The model under review builds one solid part; all positions refer to its coordinate system, in mm. A direction names the side the tool comes from. Round coordinates to 2 decimals unless told otherwise and drop trailing zeros. Write each loop counter-clockwise with the first axis right and the second up, starting at its lowest first coordinate (ties: lowest second). Pieces come first, ordered by that corner, then holes. Notation, with made-up numbers: (-27.75, 73) -> (-21.75, 73) arc R19 ccw to (-21.75, 87) -> close; hole circle Ø6 at (81, 61). An arc over 180 degrees is marked (long way). Use CSV: the item, a comma, the result in double quotes. Start each with the question number.
1) For pin 1 Ø3 at (y, z) = (-23, 26.5) entering from -X; pin 2 Ø5 at (x, z) = (-10, -15) entering from +Y; pin 3 Ø6 at (x, y) = (11.5, 27.5) entering from -Z; pin 4 Ø6.5 at (x, y) = (6.4, -11.09) entering from -Z, all flat-tipped, find the tip position at first contact; note any pin that passes through.
2) Take a section at A-A, the plane y = -9.5. State how many separate pieces and enclosed holes the cut face has, then the cut area to 3 significant figures.
3) Wall thickness on probe 1 along Z at (x, y) = (6, -2.5); probe 2 along Z at (x, y) = (-1, -24.5); probe 3 along X at (y, z) = (-18, 4.5): over which ranges is each line inside the solid? List them lowest first. Write a range as [from, to].
4) Machinability: for faces 1 (the face through (-0.867, 3.905, -20.514)), 2 (the face through (-4.336, -19.524, -3.853)), 3 (the face through (-4.336, -19.524, 44.854)), which of the approach directions +Z, -Z, +X, -X, +Y, -Y give a long, thin tool a straight path to every point of the face, cutting with its end or side? Answer none if there is none.
5) Mouldability with a two-part tool opening along X and no side actions: class faces 4 (the face through (15.213, -4.791, -23.021)), 5 (the face through (-10, 0, -23)), 6 (the face through (3, 3, -19.5)), 7 (the face through (5.11, 8.6, -23.02)) as released by +X, released by -X, zero draft, split by the parting line, or undercut.
6) Take a section at B-B, the plane z = 17. Give the boundary of the cut face in (x, y).
from build123d import *

# Parameters (mm, degrees)
SKETCH_1_R          = 35.1
EXTRUDE_1_DEPTH     = 45.1
SKETCH_3_R          = 30
SKETCH_3_R_2        = 20
EXTRUDE_2_DEPTH     = 3.5
SKETCH_3_4_R        = 20
EXTRUDE_3_DEPTH     = 24.5
FILLET_1_R          = 5
FILLET_2_R          = 20
FILLET_3_R          = 1
SKETCH_6_R          = 2.8
CUT_EXTRUDE_1_DEPTH = 4
SKETCH_7_R          = 25
SKETCH_7_R_2        = 20
CUT_EXTRUDE_2_DEPTH = 0.5


with BuildPart() as part:
    # Sketch 1 → Extrude 1 (new body)
    with BuildSketch(Plane.XY):
        Circle(SKETCH_1_R)
    extrude(amount=EXTRUDE_1_DEPTH)

    # Sketch 3 → Extrude 2 (add)
    with BuildSketch(Plane.XY):
        Circle(SKETCH_3_R)
        Circle(SKETCH_3_R_2, mode=Mode.SUBTRACT)
    extrude(amount=-EXTRUDE_2_DEPTH)

    # Sketch 3_4 → Extrude 3 (add)
    with BuildSketch(Plane.XY):
        Circle(SKETCH_3_4_R)
    extrude(amount=-EXTRUDE_3_DEPTH)

    # Sketch 4 → Cut-Revolve 2 (revolve, cut)
    with BuildSketch(Plane(origin=(0, 0, 0), x_dir=(1, 0, 0), z_dir=(0, 1, 0)), mode=Mode.PRIVATE) as cut_revolve_2_sk:
        Polygon((-15.95, 24.5), (-20, 24.5), (-20, 7.5), (-15.95, 19.5), (-4, 19.5), (-4, 21.5), (-15.95, 21.5), align=None)
    revolve(cut_revolve_2_sk.sketch.rotate(Axis((0, 0, -24.5), (0, 0, -1)), 180), axis=Axis((0, 0, -24.5), (0, 0, -1)), mode=Mode.SUBTRACT)

    # Fillet 1
    fillet_1_edges = [part.edges().sort_by_distance(p)[0] for p in [
        (-35.1, 0, 0),
        (-35.1, 0, 45.1),
    ]]
    fillet(fillet_1_edges, radius=FILLET_1_R)

    # Fillet 2
    fillet_2_edges = [part.edges().sort_by_distance(p)[0] for p in [
        (-20, 0, -7.5),
    ]]
    fillet(fillet_2_edges, radius=FILLET_2_R)

    # Fillet 3
    fillet_3_edges = [part.edges().sort_by_distance(p)[0] for p in [
        (-30, 0, -3.5),
    ]]
    fillet(fillet_3_edges, radius=FILLET_3_R)

    # Sketch 6 → Cut-Extrude 1 (cut)
    with BuildSketch(Plane(origin=(0, 0, -24.5), x_dir=(-1, 0, 0), z_dir=(0, 0, -1))):
        with Locations((12.8, 0)):
            Circle(SKETCH_6_R)
        with Locations((-6.4, -11.085125168)):
            Circle(SKETCH_6_R)
        with Locations((-6.4, 11.085125168)):
            Circle(SKETCH_6_R)
    extrude(amount=-CUT_EXTRUDE_1_DEPTH, mode=Mode.SUBTRACT)

    # Sketch 7 → Cut-Extrude 2 (cut)
    with BuildSketch(Plane.XY.offset(45.1)):
        Circle(SKETCH_7_R)
        Circle(SKETCH_7_R_2, mode=Mode.SUBTRACT)
    extrude(amount=-CUT_EXTRUDE_2_DEPTH, mode=Mode.SUBTRACT)


solid = part.part
Values found:
1,pin 1,"x = -27.74"
1,pin 2,"y = 16.1"
1,pin 3,"z = -3.5"
1,pin 4,"z = -24.5"
2,separate pieces,"3"
2,enclosed holes,"0"
2,area,"3,790 mm²"
3,probe 1,"[-24.5, -21.5], [-19.5, 45.1]"
3,probe 2,"[-3.5, 44.6]"
3,probe 3,"[-30.1, 30.1]"
4,face 1,"none"
4,face 2,"-Z"
4,face 3,"+Z"
5,face 4,"split by the parting line"
5,face 5,"undercut"
5,face 6,"zero draft"
5,face 7,"undercut"
6,outline,"circle Ø70.2 at (0, 0)"
